Autodesk Inventor part; units mm, degrees
ref_plane "YZ Plane" through (0, 0, 0) normal (1, 0, 0) x (0, 1, 0)
ref_plane "XZ Plane" through (0, 0, 0) normal (0, 1, 0) x (-1, 0, 0)
ref_plane "XY Plane" through (0, 0, 0) normal (0, 0, 1) x (1, 0, 0)
sketch "Sketch1" plane through (0, 0, 0) normal (0, 1, 0) x (-1, 0, 0)
  circle A0 centre (0, 0) radius 1.6
  circle A1 centre (0, 0) radius 3.8
  dimension "d0" = 3.2
  dimension "d1" = 2.2
extrude "Extrusion1" add sketch "Sketch1" along normal mid plane 4.7
fillet "Fillet1" radius 0.2 2 edges at (1.6, 2.35, 0) (1.6, -2.35, 0)
properties part number "Soportes tarjeta conectora CAEN"
Can you work these out from the model? Positions are in its coordinate system, mm. Round coordinates to 2 decimals unless told otherwise and drop trailing zeros. Write each loop counter-clockwise with the first axis right and the second up, starting at its lowest first coordinate (ties: lowest second). Pieces come first, ordered by that corner, then holes. Notation, with made-up numbers: M 63.25,85.25 L 71.25,85.25 A27 cw 71.25,115.25 Z; hole C 81,42 d10. An arc over 180 degrees is marked long. Use CSV: the item, a comma, the result in double quotes.
(1) We'd pull the mould along X, two halves only. Please class faces 1 (the cylindrical face through (3.796, -0.033, -0.167)), 2 (the flat face through (-2, 2.35, -1)), 3 (the cylindrical face through (1.27, -0.03, 0.97)): +X half, -X half, draft (parallel to the pull), parting line (faces both ways), or undercut.
Check values:
face 1,"parting line"
face 2,"draft"
face 3,"undercut"
(2) Imagine slicing it at A-A (z = 0). Write out the boundary of the cut face in (x, y), plus the area to 3 significant figures.
Check values:
outline,"M -3.8,-2.35 L -1.8,-2.35 A0.2 ccw -1.6,-2.15 L -1.6,2.15 A0.2 ccw -1.8,2.35 L -3.8,2.35 Z; M 1.6,-2.15 A0.2 ccw 1.8,-2.35 L 3.8,-2.35 L 3.8,2.35 L 1.8,2.35 A0.2 ccw 1.6,2.15 Z"
area,"20.6 mm^2"
(3) I need wall thicknesses on line 1 along Z through (x, y) = (0, -0.15); line 2 along Z through (x, y) = (0.5, 0.7). Which ranges of each line are inside material? Lowest first, please.
Check values:
line 1,"-3.8 to -1.6, 1.6 to 3.8"
line 2,"-3.77 to -1.52, 1.52 to 3.77"
(4) Imagine slicing it at C-C (y = -0.65). Write out the boundary of the cut face in (x, z), plus the area to 3 significant figures.
Check values:
outline,"C 0,0 d7.6; hole C 0,0 d3.2"
area,"37.3 mm^2"
(5) I'm going to push flat-ended pins straight in: pin 1 (1 mm diameter, centred on x = -2, y = -0.5, fed in from +Z); pin 2 (1.5 mm diameter, centred on x = 1.5, y = -1, fed in from +Z); pin 3 (3 mm diameter, centred on x = 0, z = 0, fed in from +Y). Where does each tip first touch, or does it pass through?
Check values:
pin 1,"z = 3.49"
pin 2,"z = 3.73"
pin 3,"through"
(6) Imagine slicing it at B-B (x = 0). Write out the boundary of the cut face in (y, z).
Check values:
outline,"M -2.35,-3.8 L 2.35,-3.8 L 2.35,-1.8 A0.2 ccw 2.15,-1.6 L -2.15,-1.6 A0.2 ccw -2.35,-1.8 Z; M -2.35,1.8 A0.2 ccw -2.15,1.6 L 2.15,1.6 A0.2 ccw 2.35,1.8 L 2.35,3.8 L -2.35,3.8 Z"
(7) Imagine slicing it at D-D (z = -2.75). Write out the boundary of the cut face in (x, y).
Check values:
outline,"M -2.62,-2.35 L 2.62,-2.35 L 2.62,2.35 L -2.62,2.35 Z"
